Geometry check sheet. Reference: the model listing, model coordinates, mm. Coordinates: 2 decimals unless noted, no trailing zeros. Loops run counter-clockwise (first coordinate to the right, second up) from the corner with the lowest first, then second, coordinate; pieces in that order, holes last.
from build123d import *

# Parameters (mm, degrees)
ESQUISSE1_W             = 91
ESQUISSE1_H             = 77
BOSS_EXTRU_1_DEPTH      = 1.2
ESQUISSE2_W             = 85.996652656
ESQUISSE2_H             = 63.887239855
ENL_V_MAT_EXTRU_1_DEPTH = 0.2
ESQUISSE3_W             = 17.000934191
ESQUISSE3_H             = 1.101570178
ENL_V_MAT_EXTRU_2_DEPTH = 0.2


with BuildPart() as part:
    # Esquisse1 → Boss.-Extru.1 (new body)
    with BuildSketch(Plane.XY):
        with Locations((45.5, 38.5)):
            Rectangle(ESQUISSE1_W, ESQUISSE1_H)
    extrude(amount=BOSS_EXTRU_1_DEPTH)

    # Esquisse2 → Enlèv. mat.-Extru.1 (cut)
    with BuildSketch(Plane.XY.offset(1.2)):
        with Locations((45.498164964, 42.446254928)):
            Rectangle(ESQUISSE2_W, ESQUISSE2_H)
    extrude(amount=-ENL_V_MAT_EXTRU_1_DEPTH, mode=Mode.SUBTRACT)

    # Esquisse3 → Enlèv. mat.-Extru.2 (cut)
    with BuildSketch(Plane.XY.offset(1.2)):
        with Locations((45.496546397, 2.848297653)):
            Rectangle(ESQUISSE3_W, ESQUISSE3_H)
    extrude(amount=-ENL_V_MAT_EXTRU_2_DEPTH, mode=Mode.SUBTRACT)


solid = part.part
1) Material ranges on probe 1 along Y at (x, z) = (17, 1.05); probe 2 along X at (y, z) = (22, 1.05); probe 3 along Z at (x, y) = (70, 71), recorded low to high.
Data:
probe 1: y = 0 to 10.5, 74.39 to 77
probe 2: x = 0 to 2.5, 88.5 to 91
probe 3: z = 0 to 1
2) Section check A-A on x = 46.5. Record the cut outline in (y, z).
Data:
outline: (0, 0) - (77, 0) - (77, 1.2) - (74.39, 1.2) - (74.39, 1) - (10.5, 1) - (10.5, 1.2) - (3.4, 1.2) - (3.4, 1) - (2.3, 1) - (2.3, 1.2) - (0, 1.2) - close
3) Section check C-C on x = 80. Record the cut outline in (y, z).
Data:
outline: (0, 0) - (77, 0) - (77, 1.2) - (74.39, 1.2) - (74.39, 1) - (10.5, 1) - (10.5, 1.2) - (0, 1.2) - close
4) Depth check by flat-ended pin: pin 1 (2 mm diameter, centred on x = 16, y = 54.5, fed in from +Z). Enter the tip coordinate at first touch or a pass-through.
Data:
pin 1: stops at z = 1
5) Mould release check, pull along X, two halves, no side actions. Record for faces 1 (the flat face through (45, 43, 1)), 2 (the flat face through (45, 39, 0)): +X half, -X half, draft (parallel to the pull), parting line (faces both ways), or undercut.
Data:
face 1: undercut
face 2: draft
6) Section check B-B on y = 54. Record the cut outline in (x, z).
Data:
outline: (0, 0) - (91, 0) - (91, 1.2) - (88.5, 1.2) - (88.5, 1) - (2.5, 1) - (2.5, 1.2) - (0, 1.2) - close
